Autodesk Fusion 360 part; units mm, degrees
sketch "Sketch1" plane through (0, 0, 0) normal (0, 0, 1) x (1, 0, 0)
  circle A0 centre (13.3357, 19.0453) radius 5
  circle A1 centre (13.3357, -19.0453) radius 5
  line L0 (0, 0) -> (80.5902, 0) construction
  line L1 (0, 0) -> (13.3357, 19.0453) construction
  arc A2 (10.4678, 14.9495) -> (10.4678, -14.9495) centre (0, 0) ccw
  arc A3 (9.5367, 22.2961) -> (9.5367, -22.2961) centre (0, 0) ccw
  line L2 (-13.7136, 20) -> (-56.7136, 20)
  line L3 (-56.7136, -20) -> (-13.7136, -20)
  line L4 (0, 0) -> (-230.6085, 0) construction
  circle A4 centre (13.3357, 19.0453) radius 2
  circle A5 centre (13.3357, -19.0453) radius 2
  line L5 (-63.7136, 13) -> (-63.7136, -13)
  arc A6 (-56.7136, 20) -> (-63.7136, 13) centre (-56.7136, 13) ccw
  arc A7 (-63.7136, -13) -> (-56.7136, -20) centre (-56.7136, -13) ccw
  circle A8 centre (-56.7136, 13) radius 2
  circle A9 centre (-56.7136, -13) radius 2
  circle A10 centre (-36.7136, 13) radius 2
  circle A11 centre (-36.7136, -13) radius 2
  point P0 (-63.7136, 20)
  point P1 (-63.7136, -20)
  dimension "d1" = 36.5
  dimension "d2" = 6
  dimension "d3" = 55
  dimension "d4" = 10
  dimension "d5" = 40
  dimension "d23" = 4
  dimension "d25" = 50
  dimension "d26" = 7
  dimension "d27" = 4
  dimension "d30" = 20
extrude "Extrude1" add sketch "Sketch1" along normal blind 4
fillet "Fillet1" radius 10 4 edges at (9.5367, 22.2961, 2) (-13.7136, 20, 2) (9.5367, -22.2961, 2) (-13.7136, -20, 2)
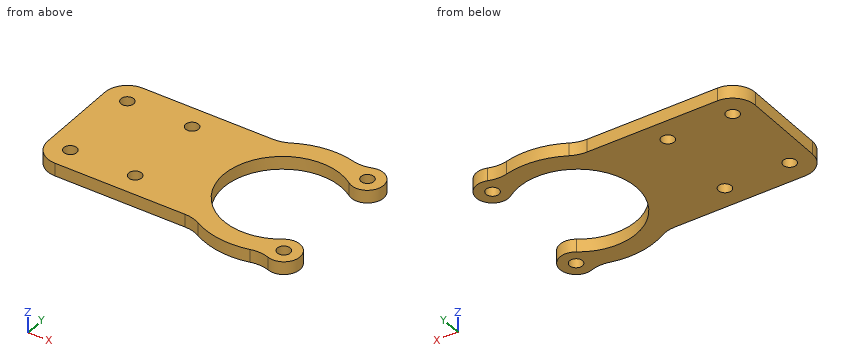
The model under review builds one solid part; all positions refer to its coordinate system, in mm. Give positions to 0.01 mm unless a question says otherwise; leave off trailing zeros. Order: outer loops, then holes, each group sorted by start corner. A loop starts at its lowest first (then second) coordinate and runs counter-clockwise, first axis right, second up. Notation, with made-up numbers: M 77,-33.75 L 103,-33.75 A24 ccw 103,-21.75 Z; hole C -22,50.25 d10. An arc over 180 degrees is marked long. Answer in a Markdown table with one row per item. Add a question column.
1. Add section C-C on y = 0. State the section outline as (x, z) points, plus the area to 3 significant figures.
2. To check wall thickness, follow line 1 along Y through (x, z) = (0, 2.65); line 2 along Y through (x, z) = (-58.5, 3.2); line 3 along Y through (x, z) = (-56, 1.7). State the ranges of each line that lie inside material, in increasing order.
3. For pin 1 Ø2 at (x, z) = (-44, 1) entering from +Y; pin 2 Ø1 at (y, z) = (-8.5, 3.5) entering from +X, all flat-tipped, find the tip position at first contact; note any pin that passes through.
4. Add section D-D on x = -49. State the section outline as (y, z) points.
5. Add section B-B on x = 12.5. State the section outline as (y, z) points.
6. Add section A-A on x = 0. State the section outline as (y, z) points.
The answers:
| question | item | result |
|---|---|---|
| 1 | outline | M -63.71,0 L -18.25,0 L -18.25,4 L -63.71,4 Z |
| 1 | area | 182 mm2 |
| 2 | line 1 | -24.25 to -18.25, 18.25 to 24.25 |
| 2 | line 2 | -19.77 to -13.9, -12.1 to 12.1, 13.9 to 19.77 |
| 2 | line 3 | -20 to -14.87, -11.13 to 11.13, 14.87 to 20 |
| 3 | pin 1 | y = 20 |
| 3 | pin 2 | x = -15.88 |
| 4 | outline | M -20,0 L 20,0 L 20,4 L -20,4 Z |
| 5 | outline | M -23.97,0 L -20.86,0 L -20.86,4 L -23.97,4 Z; M -17.23,0 L -14.12,0 L -14.12,4 L -17.23,4 Z; M 14.12,0 L 17.23,0 L 17.23,4 L 14.12,4 Z; M 20.86,0 L 23.97,0 L 23.97,4 L 20.86,4 Z |
| 6 | outline | M -24.25,0 L -18.25,0 L -18.25,4 L -24.25,4 Z; M 18.25,0 L 24.25,0 L 24.25,4 L 18.25,4 Z |
